Model file for the job. Use its own axes, mm. Face numbers are marked on the shaded views. Round coordinates to 2 decimals unless told otherwise and drop trailing zeros. Order: outer loops, then holes, each group sorted by start corner. A loop starts at its lowest first (then second) coordinate and runs counter-clockwise, first axis right, second up. Notation, with made-up numbers: (33, 84.5) -> (78, 84.5) arc R22 cw to (78, 105.5) -> close; hole circle Ø6 at (-9.75, 83). An arc over 180 degrees is marked (long way). Put each result on its own line as item: value. Start each with the question number.
Q1. Cut at C-C, the plane z = -25.5. List the corners of the cut face in (x, y).
Q2. Pull direction X, two halves, no side cores. Call the marked faces 1, 2 and 3: released by +X, released by -X, zero draft, split by the parting line, or undercut.
Q3. Cut at B-B, the plane x = 13. List the corners of the cut face in (y, z), and give its area (3 significant figures).
Q4. Flat gauge pins, fed straight in: P1, Ø7.5, axis at y = 69, z = -4.5, coming from the -X side; P2, Ø4, axis at x = 3.5, y = 108, coming from the +Z side (3 decimals); P3, Ø5, axis at x = 20.5, z = -8, coming from the +Y side; P4, Ø9, axis at y = 111, z = -3.5, coming from the -X side (3 decimals). Where does each tip first touch, or does it go through?
Q5. Cut at D-D, the plane x = 27. List the corners of the cut face in (y, z), and give its area (3 significant figures).
Q6. Probe L1, parallel to Z at x = 6.5, y = 146.5 (3 decimals); L2, parallel to X at y = 143.5, z = -6.5 (3 decimals); L3, parallel to Y at x = 18, z = -16. List the from-to ranges inside material, lowest first.
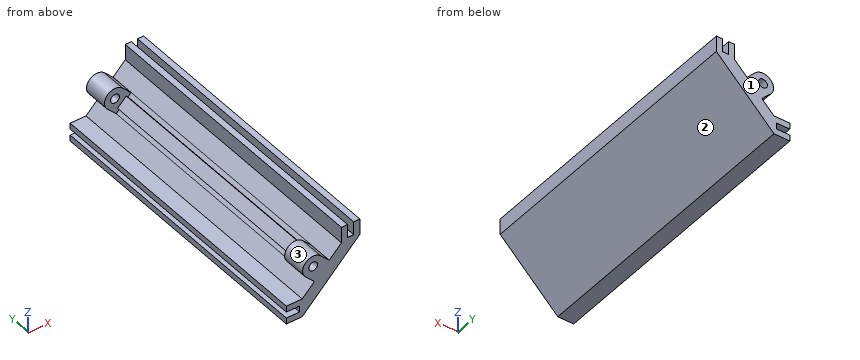
from build123d import *

# Parameters (mm, degrees)
SKETCH1_R           = 2.286
BOSS_EXTRUDE1_DEPTH = 152.4
SKETCH2_W           = 10.922
SKETCH2_H           = 127
CUT_EXTRUDE1_DEPTH  = 11.811
SKETCH3_W           = 6.35
SKETCH3_H           = 127
BOSS_EXTRUDE2_DEPTH = 1.27


with BuildPart() as part:
    # Sketch1 → Boss-Extrude1 (new body)
    with BuildSketch(Plane(origin=(0, 0, 0), x_dir=(1, 0, 0), z_dir=(0, 1, 0))):
        with BuildLine():
            Line((38.1, 0), (38.1, 8.209871939))
            Line((38.1, 8.209871939), (8.209871939, 38.1))
            Line((8.209871939, 38.1), (0, 38.1))
            Line((0, 38.1), (0, 34.925))
            Line((0, 34.925), (6.858, 34.925))
            Line((6.858, 34.925), (6.858, 31.75))
            Line((6.858, 31.75), (0, 31.75))
            Line((0, 31.75), (0, 28.575))
            Line((0, 28.575), (8.209871939, 28.575))
            Line((8.209871939, 28.575), (14.530925838, 22.253946102))
            Line((14.530925838, 22.253946102), (10.040797777, 17.763818041))
            ThreePointArc((10.040797777, 17.763818041), (10.040797777, 10.040797777), (17.763818041, 10.040797777))
            Line((17.763818041, 10.040797777), (22.253946102, 14.530925838))
            Line((22.253946102, 14.530925838), (28.575, 8.209871939))
            Line((28.575, 8.209871939), (28.575, 0))
            Line((28.575, 0), (31.75, 0))
            Line((31.75, 0), (31.75, 6.858))
            Line((31.75, 6.858), (34.925, 6.858))
            Line((34.925, 6.858), (34.925, 0))
            Line((34.925, 0), (38.1, 0))
        make_face()
        with Locations((13.902307909, 13.902307909)):
            Circle(SKETCH1_R, mode=Mode.SUBTRACT)
    extrude(amount=BOSS_EXTRUDE1_DEPTH)

    # Sketch2 → Cut-Extrude1 (cut)
    with BuildSketch(Plane(origin=(18.39243597, 0, -18.39243597), x_dir=(0.707106781, 0, 0.707106781), z_dir=(-0.707106781, 0, 0.707106781))):
        with Locations((0, 76.2)):
            Rectangle(SKETCH2_W, SKETCH2_H)
    extrude(amount=CUT_EXTRUDE1_DEPTH, mode=Mode.SUBTRACT)

    # Sketch3 → Boss-Extrude2 (add)
    with BuildSketch(Plane(origin=(18.39243597, 0, -18.39243597), x_dir=(0.707106781, 0, 0.707106781), z_dir=(-0.707106781, 0, 0.707106781))):
        with Locations((0, 76.2)):
            Rectangle(SKETCH3_W, SKETCH3_H)
    extrude(amount=BOSS_EXTRUDE2_DEPTH)


solid = part.part
Ans:
1. outline: (11.28, 0) -> (20.81, 0) -> (20.81, 152.4) -> (11.28, 152.4) -> close
2. face 1: zero draft
2. face 2: released by +X
2. face 3: undercut
3. outline: (0, -33.31) -> (152.4, -33.31) -> (152.4, -23.78) -> (0, -23.78) -> close; (0, -20.72) -> (12.7, -20.72) -> (12.7, -16) -> (0, -16) -> close; (0, -11.8) -> (12.7, -11.8) -> (12.7, -8.52) -> (0, -8.52) -> close; (139.7, -20.72) -> (152.4, -20.72) -> (152.4, -16) -> (139.7, -16) -> close; (139.7, -11.8) -> (152.4, -11.8) -> (152.4, -8.52) -> (139.7, -8.52) -> close
3. area: 1,650 mm^2
4. P1: stops at x = 28.53
4. P2: stops at z = -28.575
4. P3: passes through
4. P4: stops at x = 28.575
5. outline: (0, -19.31) -> (152.4, -19.31) -> (152.4, -9.78) -> (0, -9.78) -> close
5. area: 1,450 mm^2
6. L1: z = -38.1 to -34.925, -31.75 to -28.575
6. L2: x = 28.575 to 31.75, 34.925 to 38.1
6. L3: y = 0 to 12.7, 139.7 to 152.4
